Study the drawing (mm; zero at the part's minimum x, y, z) and answer. A direction names the side the tool comes from. Give positions to 0.01 mm unless a question says otherwise; leave off trailing zeros. Write each loop counter-clockwise with the first axis right and the second up, starting at its lowest first coordinate (ties: lowest second). Pieces come first, ordered by that corner, then holes. Notation, with made-up numbers: (4.5, -8) - (13.5, -8) arc R23 cw to (13.5, 21) - close; hole circle Ø10 at (41.5, 42.5). An arc over 180 degrees is marked (long way). One line per item, written item: value. Start each with the question number.
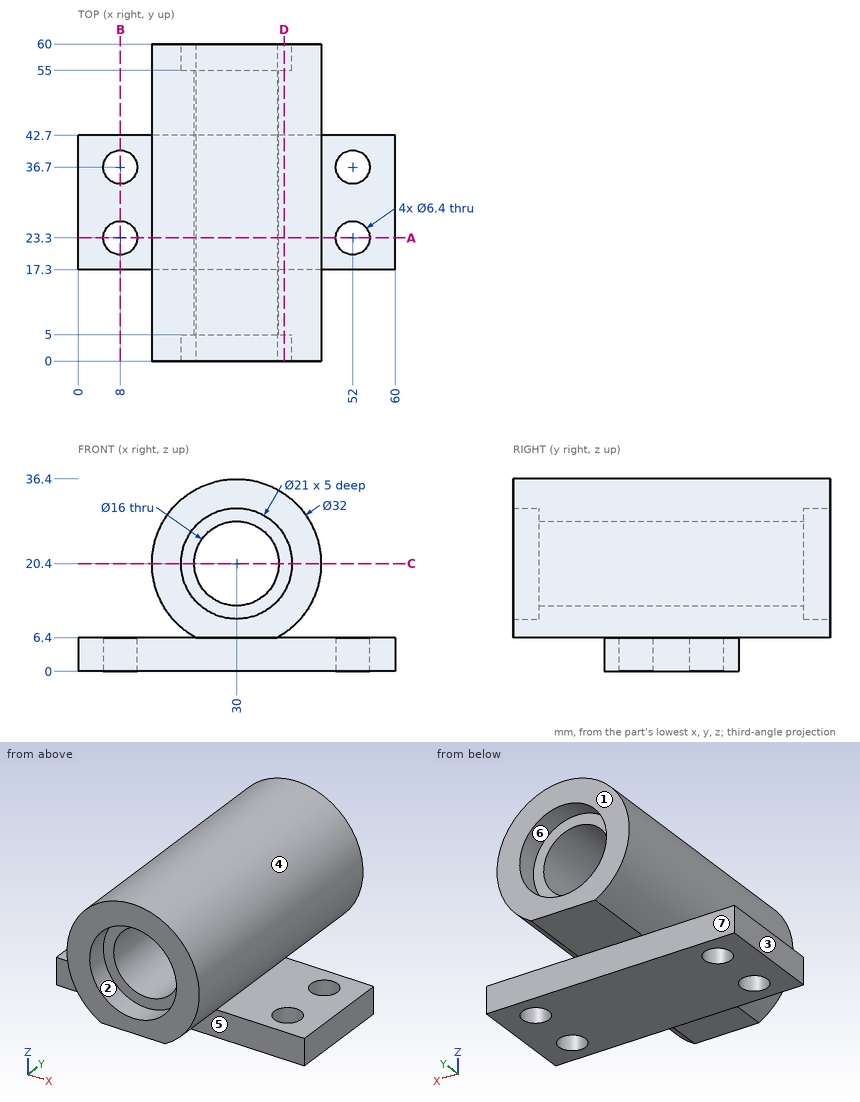
Item 1: The mould has two halves that part along X. Classify the marked faces 1, 2, 3 and 4: +X half, -X half, draft (parallel to the pull), parting line (faces both ways), or undercut.
Item 2: For the marked faces 5, 6 and 7, determine the directions among +Z, -Z, +X, -X, +Y, -Y from which every point of the face is accessible in a straight line to the end or side of a thin tool.
Item 3: Find section D-D on x = 39. Determine the outline of the cut face in (y, z), plus the area to 3 significant figures.
Item 4: Straight lines are drawn through the part: line 1 along Y through (x, z) = (8, 3.5); line 2 along Y through (x, z) = (6, 5.5); line 3 along Z through (x, y) = (31.5, 18.5). For each, find the intervals that lie inside material, in ascending order.
Item 5: Each of these flat-tipped pins is pushed along its axis until it touches: pin 1 Ø10 at (x, y) = (15.5, 52.5) entering from +Z; pin 2 Ø3 at (y, z) = (11.5, 15.5) entering from +X; pin 3 Ø6 at (x, z) = (36.5, 20.5) entering from -Y; pin 4 Ø6 at (x, y) = (8, 23.3) entering from +Z. Where does it stop, or does it pass through?
Item 6: Find section B-B on x = 8. Determine the outline of the cut face in (y, z), plus the area to 3 significant figures.
Item 7: Find section A-A on y = 23.3. Determine the outline of the cut face in (x, z).
Item 8: Find section C-C on z = 20.4. Determine the outline of the cut face in (x, y), plus the area to 3 significant figures.
Values:
1. face 1: draft
1. face 2: undercut
1. face 3: -X half
1. face 4: parting line
2. face 5: -Z, +X, -X, -Y
2. face 6: +Y
2. face 7: -Z, +X, -X, +Y
3. outline: (0, 7.17) - (60, 7.17) - (60, 14.99) - (55, 14.99) - (55, 25.81) - (60, 25.81) - (60, 33.63) - (0, 33.63) - (0, 25.81) - (5, 25.81) - (5, 14.99) - (0, 14.99) - close; (17.3, 0) - (42.7, 0) - (42.7, 6.4) - (17.3, 6.4) - close
3. area: 1,640 mm^2
4. line 1: 17.3 to 20.1, 26.5 to 33.5, 39.9 to 42.7
4. line 2: 17.3 to 20.8, 25.8 to 34.2, 39.2 to 42.7
4. line 3: 0 to 12.54, 28.26 to 36.33
5. pin 1: z = 33.27
5. pin 2: x = 45.63
5. pin 3: y = 5
5. pin 4: through
6. outline: (17.3, 0) - (20.1, 0) - (20.1, 6.4) - (17.3, 6.4) - close; (26.5, 0) - (33.5, 0) - (33.5, 6.4) - (26.5, 6.4) - close; (39.9, 0) - (42.7, 0) - (42.7, 6.4) - (39.9, 6.4) - close
6. area: 80.6 mm^2
7. outline: (0, 0) - (4.8, 0) - (4.8, 6.4) - (0, 6.4) - close; (11.2, 0) - (48.8, 0) - (48.8, 6.4) - (37.75, 6.4) arc R16 ccw (long way) to (22.25, 6.4) - (11.2, 6.4) - close; (55.2, 0) - (60, 0) - (60, 6.4) - (55.2, 6.4) - close; hole circle Ø16 at (30, 20.4)
8. outline: (14, 0) - (19.5, 0) - (19.5, 5) - (22, 5) - (22, 55) - (19.5, 55) - (19.5, 60) - (14, 60) - close; (38, 5) - (40.5, 5) - (40.5, 0) - (46, 0) - (46, 60) - (40.5, 60) - (40.5, 55) - (38, 55) - close
8. area: 910 mm^2
